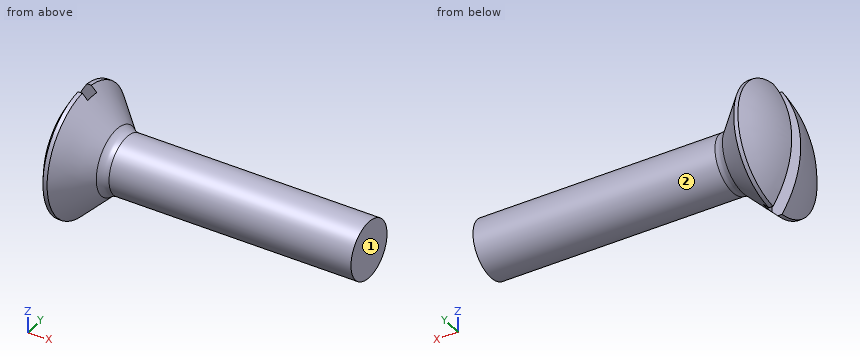
```python
from build123d import *

# Parameters (mm, degrees)
SLOT_DEPTH      = 12.1041235
SLOT_DEPTH_BACK = 12.1041235
SKE_SLOT_W      = 1
SKE_SLOT_H      = 0.5


with BuildPart() as part:
    # Ske-Screw → Base (revolve)
    with BuildSketch(Plane.XY, mode=Mode.PRIVATE) as base_sk:
        with BuildLine():
            Line((0.659341382, 2.2), (0.805787992, 2.2))
            Line((0.805787992, 2.2), (1.859341382, 1.146446609))
            ThreePointArc((1.859341382, 1.146446609), (2.021553057, 1.038060234), (2.212894773, 1))
            Line((2.212894773, 1), (10.659341382, 1))
            Line((10.659341382, 1), (10.659341382, 0))
            Line((10.659341382, 0), (0.659341382, 0))
            Line((0.659341382, 0), (0, 0))
            ThreePointArc((0, 0), (0.168379294, 1.148339133), (0.659341382, 2.2))
        make_face()
    revolve(base_sk.sketch.rotate(Axis((-1.349906986, 0, 0), (1, 0, 0)), 90), axis=Axis((-1.349906986, 0, 0), (1, 0, 0)))

    # Ske-Slot → Slot (cut, two sides: drawn at the far end of the back side and taken through both)
    with BuildSketch(Plane.XY.offset(-SLOT_DEPTH_BACK)):
        with Locations((0.5, 0)):
            Rectangle(SKE_SLOT_W, SKE_SLOT_H)
    extrude(amount=SLOT_DEPTH + SLOT_DEPTH_BACK, mode=Mode.SUBTRACT)


solid = part.part
```
Input: part model. Units: mm. Frame: model coordinates. Face numbers are marked on the shaded views. A direction names the side the tool comes from. Round coordinates to 2 decimals unless told otherwise and drop trailing zeros. Loops run counter-clockwise (first coordinate to the right, second up) from the corner with the lowest first, then second, coordinate; pieces in that order, holes last.
1) Section query C-C on x = 4.25. Return the cut outline in (y, z), plus the area to 3 significant figures.
Ans:
outline: circle Ø2 at (0, 0)
area: 3.14 mm2
2) Section query A-A on z = 0. Return the cut outline in (x, y), plus the area to 3 significant figures.
Ans:
outline: (0.01, -0.25) arc R4 ccw to (0.66, -2.2) - (0.81, -2.2) - (1.86, -1.15) arc R0.5 cw to (2.21, -1) - (10.66, -1) - (10.66, 1) - (2.21, 1) arc R0.5 cw to (1.86, 1.15) - (0.81, 2.2) - (0.66, 2.2) arc R4 ccw to (0.01, 0.25) - (1, 0.25) - (1, -0.25) - close
area: 23.3 mm2
3) Pin query (flat end, axial travel): pin 1 (1 mm diameter, centred on x = 4.5, z = -1, fed in from +Y); pin 2 (1.1 mm diameter, centred on x = 0.5, z = -0.5, fed in from -Y); pin 3 (2 mm diameter, centred on y = -1.5, z = 1, fed in from -X). Return the tip coordinate at first contact, or that it passes through.
Ans:
pin 1: stops at y = 0.87
pin 2: stops at y = -2.2
pin 3: stops at x = 0.08
4) Section query B-B on y = 0. Return the cut outline in (x, z), plus the area to 3 significant figures.
Ans:
outline: (1, -2.01) - (1.86, -1.15) arc R0.5 cw to (2.21, -1) - (10.66, -1) - (10.66, 1) - (2.21, 1) arc R0.5 cw to (1.86, 1.15) - (1, 2.01) - close
area: 20.3 mm2
5) Section query D-D on x = 1.75. Return the cut outline in (y, z), plus the area to 3 significant figures.
Ans:
outline: circle Ø2.51 at (0, 0)
area: 4.95 mm2
6) Material intervals for line 1 (Y direction, x = 6.25, z = 0); line 2 (Y direction, x = 1.75, z = 1); line 3 (X direction, y = 1.6, z = 0.95) (3 decimals), sorted ascending.
Ans:
line 1: y = -1 to 1
line 2: y = -0.76 to 0.76
line 3: x = 0.459 to 1.145
7) Set-up query: the marked faces 1 and 2. Return all of +Z, -Z, +X, -X, +Y, -Y with unobstructed straight access to the full face (end or side cutting, diameter ignored); none if empty.
Ans:
face 1: +Z, -Z, +X, +Y, -Y
face 2: +X
